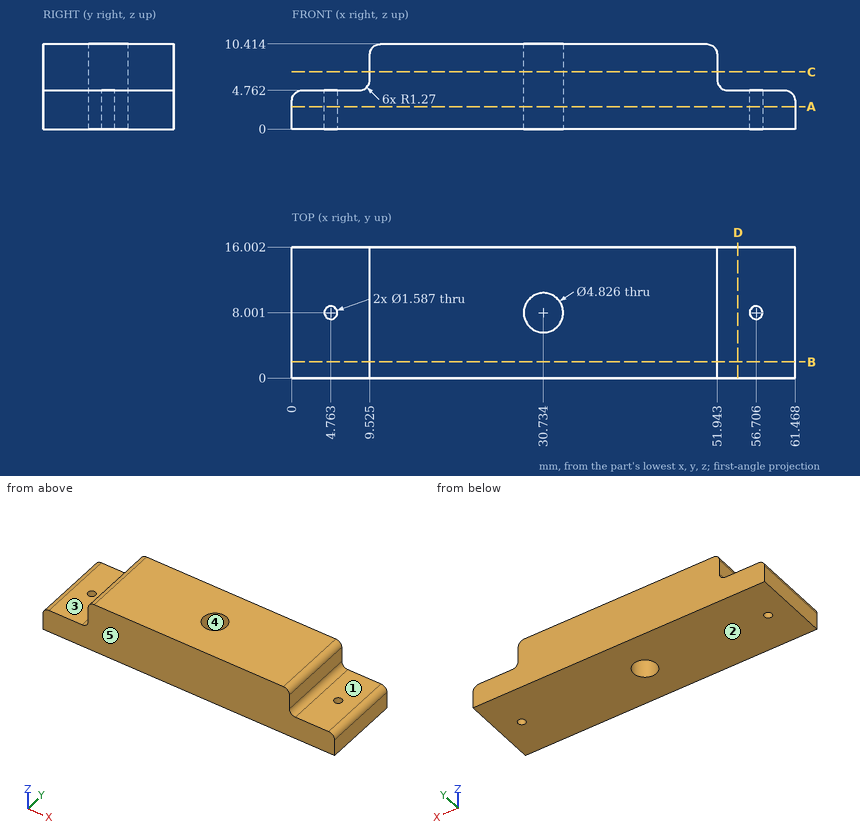
Geometry check sheet. Reference: drawing and pictorial views, mm from the part's lowest x, y, z. A direction names the side the tool comes from. Coordinates: 2 decimals unless noted, no trailing zeros. Order: outer loops, then holes, each group sorted by start corner. A loop starts at its lowest first (then second) coordinate and runs counter-clockwise, first axis right, second up. Notation, with made-up numbers: (5.25, -30.75) -> (46.25, -30.75) arc R28 cw to (46.25, -1.75) -> close; hole circle Ø10 at (-32.5, 73). An arc over 180 degrees is marked (long way). Put each result on its own line as item: value. Start each with the question number.
1) Cross-section at B-B (y = 2). Enter the section's corners in (x, z) (1 decimal), plus the area to 3 significant figures.
2) Release check for a two-part mould opening along X. For the marked faces 4 and 5 record: pulls with the +X half, pulls with the -X half, needs draft (parallel to the pull), parting line crosses it, or undercut.
3) Go/stop test with flat-tipped pins: pin 1 (1 mm diameter, centred on y = 12.5, z = 7.5, fed in from +X); pin 2 (3.5 mm diameter, centred on x = 4, y = 12, fed in from +Z); pin 3 (3.5 mm diameter, centred on y = 11.5, z = 7.5, fed in from -X); pin 4 (1.3 mm diameter, centred on x = 56.71, y = 8, fed in from -Z). Record where each tip stops, or that it passes through.
4) Cross-section at D-D (x = 54.5). Enter the section's corners in (y, z).
5) Cross-section at A-A (z = 2.75). Enter the section's corners in (x, y) (1 decimal).
6) Material ranges on L1, parallel to X at y = 9.5, z = 7.25 (1 decimal); L2, parallel to Z at x = 58, y = 3.25; L3, parallel to X at y = 10.5, z = 8.75 (1 decimal), recorded low to high.
7) Cross-section at C-C (z = 7). Enter the section's corners in (x, y) (1 decimal).
8) Tool access check on the marked faces 1, 2 and 3. Record the directions out of +Z, -Z, +X, -X, +Y, -Y that give a thin tool (end or side, any length) a straight path to the whole face; none if there is none.
Geometry check:
1. outline: (0, 0) -> (61.5, 0) -> (61.5, 3.5) arc R1.3 ccw to (60.2, 4.8) -> (53.2, 4.8) arc R1.3 cw to (51.9, 6) -> (51.9, 9.1) arc R1.3 ccw to (50.7, 10.4) -> (10.8, 10.4) arc R1.3 ccw to (9.5, 9.1) -> (9.5, 6) arc R1.3 cw to (8.3, 4.8) -> (1.3, 4.8) arc R1.3 ccw to (0, 3.5) -> close
1. area: 532 mm^2
2. face 4: undercut
2. face 5: needs draft
3. pin 1: stops at x = 51.94
3. pin 2: stops at z = 4.76
3. pin 3: stops at x = 9.49
3. pin 4: passes through
4. outline: (0, 0) -> (16, 0) -> (16, 4.76) -> (0, 4.76) -> close
5. outline: (0, 0) -> (61.5, 0) -> (61.5, 16) -> (0, 16) -> close; hole circle Ø1.6 at (4.8, 8); hole circle Ø4.8 at (30.7, 8); hole circle Ø1.6 at (56.7, 8)
6. L1: x = 9.5 to 28.8, 32.6 to 51.9
6. L2: z = 0 to 4.76
6. L3: x = 9.5 to 51.9
7. outline: (9.5, 0) -> (51.9, 0) -> (51.9, 16) -> (9.5, 16) -> close; hole circle Ø4.8 at (30.7, 8)
8. face 1: +Z, +X, +Y, -Y
8. face 2: -Z, +X, -X, +Y, -Y
8. face 3: +Z, -X, +Y, -Y
